Design review of the part built by this model. Coordinates are the model's own, in mm. A direction names the side the tool comes from. Round coordinates to 2 decimals unless told otherwise and drop trailing zeros. Loops run counter-clockwise (first coordinate to the right, second up) from the corner with the lowest first, then second, coordinate; pieces in that order, holes last. Notation, with made-up numbers: M -1.5,69 L 30.5,69 A3 ccw 30.5,73 Z; hole C -38.5,34.25 d4. An arc over 180 degrees is marked long. Use a Markdown table: item, result.
from build123d import *

# Parameters (mm, degrees)
EXTRUDE_1_DEPTH     = 3
SKETCH_2_R          = 4.5
SKETCH_2_R_2        = 3
EXTRUDE_2_DEPTH     = 1.5
CUT_EXTRUDE_1_DEPTH = 3
FILLET_1_R          = 1


with BuildPart() as part:
    # 草图1 → 凸台-拉伸1 (new body)
    with BuildSketch(Plane(origin=(0, 0, 0), x_dir=(1, 0, 0), z_dir=(0, 1, 0))):
        with BuildLine():
            ThreePointArc((-1.5, 0), (0, 1.5), (1.5, 0))
            Line((1.5, 0), (12.5, 0))
            ThreePointArc((12.5, 0), (8.948638165, 8.727650027), (0.3125, 12.496093139))
            ThreePointArc((0.3125, 12.496093139), (-8.727650027, 8.948638165), (-12.5, 0))
            Line((-12.5, 0), (-1.5, 0))
        make_face()
        with BuildLine():
            Line((12.5, 0), (1.5, 0))
            ThreePointArc((1.5, 0), (0, -1.5), (-1.5, 0))
            Line((-1.5, 0), (-12.5, 0))
            ThreePointArc((-12.5, 0), (-8.727650027, -8.948638165), (0.3125, -12.496093139))
            ThreePointArc((0.3125, -12.496093139), (8.948638165, -8.727650027), (12.5, 0))
        make_face()
        with BuildLine():
            ThreePointArc((0.3125, 12.496093139), (8.948638165, 8.727650027), (12.5, 0))
            Line((12.5, 0), (90, 0))
            ThreePointArc((90, 0), (93.017879978, 7.158910532), (100.25, 9.996874512))
            Line((100.25, 9.996874512), (0.3125, 12.496093139))
        make_face()
        with BuildLine():
            Line((90, 0), (12.5, 0))
            ThreePointArc((12.5, 0), (8.948638165, -8.727650027), (0.3125, -12.496093139))
            Line((0.3125, -12.496093139), (100.25, -9.996874512))
            ThreePointArc((100.25, -9.996874512), (93.017879978, -7.158910532), (90, 0))
        make_face()
        with BuildLine():
            ThreePointArc((100.25, 9.996874512), (93.017879978, 7.158910532), (90, 0))
            Line((90, 0), (110, 0))
            ThreePointArc((110, 0), (107.158910532, 6.982120022), (100.25, 9.996874512))
        make_face()
        with BuildLine():
            Line((110, 0), (90, 0))
            ThreePointArc((90, 0), (93.017879978, -7.158910532), (100.25, -9.996874512))
            ThreePointArc((100.25, -9.996874512), (107.158910532, -6.982120022), (110, 0))
        make_face()
    extrude(amount=EXTRUDE_1_DEPTH)

    # 草图2 → 凸台-拉伸2 (add)
    with BuildSketch(Plane.XZ):
        with Locations(Location((0, 0, 0), (0, 0, 90))):
            Circle(SKETCH_2_R)
        with Locations(Location((0, 0, 0), (0, 0, 270))):
            Circle(SKETCH_2_R_2, mode=Mode.SUBTRACT)
    extrude(amount=EXTRUDE_2_DEPTH)

    # 草图3 → 切除-拉伸1 (cut)
    with BuildSketch(Plane(origin=(0, 3, 0), x_dir=(1, 0, 0), z_dir=(0, 1, 0))):
        Polygon((20, 8.002501172), (20, 0), (33, 0), (33, 7.677399562), align=None)
        Polygon((33, 0), (20, 0), (20, -8.002501172), (33, -7.677399562), align=None)
        with BuildLine():
            ThreePointArc((38.5, 8), (36.805156295, 9.487291475), (35.550618759, 7.613614157))
            Line((35.550618759, 7.613614157), (38.42825626, 7.541650728))
            ThreePointArc((38.42825626, 7.541650728), (38.481955531, 7.768034906), (38.5, 8))
        make_face()
        with BuildLine():
            Line((38.42825626, 7.541650728), (35.550618759, 7.613614157))
            ThreePointArc((35.550618759, 7.613614157), (36.9625, 6.500468823), (38.42825626, 7.541650728))
        make_face()
        with BuildLine():
            ThreePointArc((38.42825626, -7.541650728), (36.9625, -6.500468823), (35.550618759, -7.613614157))
            Line((35.550618759, -7.613614157), (38.42825626, -7.541650728))
        make_face()
        with BuildLine():
            Line((38.42825626, -7.541650728), (35.550618759, -7.613614157))
            ThreePointArc((35.550618759, -7.613614157), (36.805156295, -9.487291475), (38.5, -8))
            ThreePointArc((38.5, -8), (38.481955531, -7.768034906), (38.42825626, -7.541650728))
        make_face()
        Polygon((41, 7.477337033), (41, 0), (58, 0), (58, 7.052204158), align=None)
        Polygon((58, 0), (41, 0), (41, -7.477337033), (58, -7.052204158), align=None)
        Polygon((66, 6.852141629), (66, 0), (83, 0), (83, 6.427008754), align=None)
        Polygon((83, 0), (66, 0), (66, -6.852141629), (83, -6.427008754), align=None)
        with BuildLine():
            ThreePointArc((88.5, 0), (87, 1.5), (85.5, 0))
            Line((85.5, 0), (88.5, 0))
        make_face()
        with BuildLine():
            Line((88.5, 0), (85.5, 0))
            ThreePointArc((85.5, 0), (87, -1.5), (88.5, 0))
        make_face()
        Polygon((100, 6.001875879), (91, 6.226946225), (91, 0), (100, 0), align=None)
        Polygon((91, 0), (91, -6.226946225), (100, -6.001875879), (100, 0), align=None)
    extrude(amount=-CUT_EXTRUDE_1_DEPTH, mode=Mode.SUBTRACT)

    # 圆角1
    fillet_1_edges = [part.edges().sort_by_distance(p)[0] for p in [
        (20, 1.5, 8.002501172),
        (20, 1.5, -8.002501172),
        (33, 1.5, -7.677399562),
        (33, 1.5, 7.677399562),
        (41, 1.5, 7.477337033),
        (41, 1.5, -7.477337033),
        (58, 1.5, -7.052204158),
        (58, 1.5, 7.052204158),
        (66, 1.5, 6.852141629),
        (66, 1.5, -6.852141629),
        (83, 1.5, -6.427008754),
        (83, 1.5, 6.427008754),
        (91, 1.5, 6.226946225),
        (91, 1.5, -6.226946225),
        (100, 1.5, -6.001875879),
        (100, 1.5, 6.001875879),
    ]]
    fillet(fillet_1_edges, radius=FILLET_1_R)


solid = part.part
1. Wall thickness on line 1 along Z through (x, y) = (0, 0.8); line 2 along Y through (x, z) = (14, 2); line 3 along Z through (x, y) = (47, 2.4): over which ranges is each line inside the solid? List them lowest first. Write a range as from..to.
Check values:
| item | result |
|---|---|
| line 1 | z = -12.5..-1.5, 1.5..12.5 |
| line 2 | y = 0..3 |
| line 3 | z = -11.33..-7.33, 7.33..11.33 |
2. The part is to be moulded in two halves that separate along Z. For faces 3 (the face through (48, 0, 8)), 4 (the face through (-1.352, -0.74, 4.292)), 5 (the face through (1.5, 1.48, -0.07)), say which applies: pulls with the +Z half, pulls with the -Z half, needs draft (parallel to the pull), parting line crosses it, or undercut.
Check values:
| item | result |
|---|---|
| face 3 | needs draft |
| face 4 | parting line crosses it |
| face 5 | undercut |
3. Take a section at B-B on y = 1.15. Count the separate pieces of the cut face and the enclosed holes in it, and give its area (3 significant figures).
Check values:
| item | result |
|---|---|
| separate pieces | 1 |
| enclosed holes | 8 |
| area | 1,840 mm² |
4. Take a section at A-A on x = 37. Give the boundary of the cut face in (y, z).
Check values:
| item | result |
|---|---|
| outline | M 0,-11.58 L 3,-11.58 L 3,-9.5 L 0,-9.5 Z; M 0,-6.5 L 3,-6.5 L 3,6.5 L 0,6.5 Z; M 0,9.5 L 3,9.5 L 3,11.58 L 0,11.58 Z |
5. Machinability: for faces 1 (the face through (1.3, 0, 1.3)), 2 (the face through (33, 2, 0)), which of the approach directions +Z, -Z, +X, -X, +Y, -Y give a long, thin tool a straight path to every point of the face, cutting with its end or side? Answer none if there is none.
Check values:
| item | result |
|---|---|
| face 1 | -Y |
| face 2 | +Y, -Y |
6. Take a section at C-C on x = 87. Give the boundary of the cut face in (y, z), and give its area (3 significant figures).
Check values:
| item | result |
|---|---|
| outline | M 0,-10.33 L 3,-10.33 L 3,-1.5 L 0,-1.5 Z; M 0,1.5 L 3,1.5 L 3,10.33 L 0,10.33 Z |
| area | 53.0 mm² |
7. Take a section at D-D on x = 8.5. Give the boundary of the cut face in (y, z).
Check values:
| item | result |
|---|---|
| outline | M 0,-12.29 L 3,-12.29 L 3,12.29 L 0,12.29 Z |
8. Insertion check: pin 1 (1.5 mm diameter, centred on y = -1, z = -4, fed in from +X); pin 2 (0.9 mm diameter, centred on y = 1.5, z = -2.5, fed in from +X); pin 3 (2.5 mm diameter, centred on y = 2, z = 2, fed in from -X); pin 4 (7.5 mm diameter, centred on x = 25.5, z = 4, fed in from -Y). Each pin has a flat end and moves straight along its axis. Give the tip position at first contact, or say it passes through.
Check values:
| item | result |
|---|---|
| pin 1 | stops at x = 3.11 |
| pin 2 | stops at x = 109.79 |
| pin 3 | stops at x = -12.48 |
| pin 4 | passes through |
